Read the model definition and answer for the solid it produces. Units are mm, in the model's axes. A direction names the side the tool comes from. Give positions to 0.01 mm unless a question says otherwise; leave off trailing zeros. Loops run counter-clockwise (first coordinate to the right, second up) from the corner with the lowest first, then second, coordinate; pieces in that order, holes last. Notation, with made-up numbers: (-34.75, 89) - (0.25, 89) arc R23 ccw to (0.25, 97) - close; hole circle Ø8 at (21, 64). An arc over 180 degrees is marked (long way). Write item = value, one per line. Start each with the question number.
from build123d import *

# Parameters (mm, degrees)
SKETCH1_R                    = 150
BOSS_EXTRUDE1_DEPTH          = 75
CHAMFER1_SIZE                = 10
BOSS_EXTRUDE2_START          = -75
BOSS_EXTRUDE2_DEPTH          = 10
CHAMFER2_SIZE                = 7
BOSS_EXTRUDE3_DEPTH          = 9
BOSS_EXTRUDE4_DEPTH          = 3.5
CIRPATTERN1_COUNT            = 4
CIRPATTERN1_COPY_1_DEPTH     = 9
CIRPATTERN1_COPY_2_DEPTH     = 9
CIRPATTERN1_COPY_3_DEPTH     = 9
CIRPATTERN1_COPY_4_DEPTH     = 3.5
CIRPATTERN1_COPY_5_DEPTH     = 3.5
CIRPATTERN1_COPY_6_DEPTH     = 3.5
CHAMFER2_OF_CIRPATTERN1_SIZE = 7
CUT_EXTRUDE1_START           = -60
CUT_EXTRUDE1_DEPTH           = 60
SKETCH6_R                    = 110
BOSS_EXTRUDE5_DEPTH          = 9
BOSS_EXTRUDE5_TAPER          = 40
SKETCH7_R                    = 15
BOSS_EXTRUDE6_DEPTH          = 20


with BuildPart() as part:
    # Sketch1 → Boss-Extrude1 (new body)
    with BuildSketch(Plane(origin=(0, 0, 0), x_dir=(1, 0, 0), z_dir=(0, 1, 0))):
        with Locations(Location((0, 0, 0), (0, 0, 270))):
            Circle(SKETCH1_R)
    extrude(amount=BOSS_EXTRUDE1_DEPTH)

    # Chamfer1
    chamfer1_edges = [part.edges().sort_by_distance(p)[0] for p in [
        (0, 75, -150),
    ]]
    chamfer(chamfer1_edges, length=CHAMFER1_SIZE)

    # Sketch2 → Boss-Extrude2 (add)
    with BuildSketch(Plane(origin=(0, 75, 0), x_dir=(1, 0, 0), z_dir=(0, 1, 0)).offset(BOSS_EXTRUDE2_START)):
        with BuildLine():
            Line((-145.236875483, 37.5), (-195.236875483, 37.5))
            Line((-195.236875483, 37.5), (-195.236875483, -37.5))
            Line((-195.236875483, -37.5), (-145.236875483, -37.5))
            ThreePointArc((-145.236875483, -37.5), (-150, 0), (-145.236875483, 37.5))
        make_face()
    boss_extrude2 = extrude(amount=BOSS_EXTRUDE2_DEPTH)

    # Chamfer2
    chamfer2_edges = [part.edges().sort_by_distance(p)[0] for p in [
        (-195.236875483, 5, -37.5),
        (-195.236875483, 5, 37.5),
    ]]
    chamfer(chamfer2_edges, length=CHAMFER2_SIZE)

    # Sketch3 → Boss-Extrude3 (add)
    with BuildSketch(Plane.XY.offset(37.5)):
        Polygon((-145.236875483, 10), (-145.236875483, 65), (-170.556875483, 65), (-188.236875483, 10), align=None)
    boss_extrude3 = extrude(amount=-BOSS_EXTRUDE3_DEPTH)

    # Sketch4 → Boss-Extrude4 (add)
    with BuildSketch(Plane(origin=(0, 10, 0), x_dir=(1, 0, 0), z_dir=(0, 1, 0))):
        Polygon((-188.236875483, -21), (-183.04072306, -18), (-183.04072306, -12), (-188.236875483, -9), (-193.433027905, -12), (-193.433027905, -18), align=None)
    boss_extrude4 = extrude(amount=BOSS_EXTRUDE4_DEPTH)

    # Mirror1: Boss-Extrude3, Boss-Extrude4 across plane
    add(boss_extrude3.mirror(Plane.XY))
    add(boss_extrude4.mirror(Plane.XY))

    # CirPattern1: Boss-Extrude2, Boss-Extrude3, Boss-Extrude4 ×4 about axis
    cirpattern1_axis = Axis((0, 0, 0), (0, 1, 0))
    add([boss_extrude2.rotate(cirpattern1_axis, i * 360 / CIRPATTERN1_COUNT) for i in range(1, CIRPATTERN1_COUNT)])
    add([boss_extrude3.rotate(cirpattern1_axis, i * 360 / CIRPATTERN1_COUNT) for i in range(1, CIRPATTERN1_COUNT)])
    add([boss_extrude4.rotate(cirpattern1_axis, i * 360 / CIRPATTERN1_COUNT) for i in range(1, CIRPATTERN1_COUNT)])

    # CirPattern1 copy 1 sketch → CirPattern1 copy 1 (add)
    with BuildSketch(Plane(origin=(-37.5, 0, 0), x_dir=(0, 0, -1), z_dir=(-1, 0, 0))):
        Polygon((-145.236875483, -10), (-145.236875483, -65), (-170.556875483, -65), (-188.236875483, -10), align=None)
    extrude(amount=-CIRPATTERN1_COPY_1_DEPTH)

    # CirPattern1 copy 2 sketch → CirPattern1 copy 2 (add)
    with BuildSketch(Plane(origin=(0, 0, 37.5), x_dir=(-1, 0, 0), z_dir=(0, 0, 1))):
        Polygon((-145.236875483, -10), (-145.236875483, -65), (-170.556875483, -65), (-188.236875483, -10), align=None)
    extrude(amount=-CIRPATTERN1_COPY_2_DEPTH)

    # CirPattern1 copy 3 sketch → CirPattern1 copy 3 (add)
    with BuildSketch(Plane(origin=(37.5, 0, 0), x_dir=(0, 0, 1), z_dir=(1, 0, 0))):
        Polygon((-145.236875483, -10), (-145.236875483, -65), (-170.556875483, -65), (-188.236875483, -10), align=None)
    extrude(amount=-CIRPATTERN1_COPY_3_DEPTH)

    # CirPattern1 copy 4 sketch → CirPattern1 copy 4 (add)
    with BuildSketch(Plane(origin=(0, 10, 0), x_dir=(0, 0, -1), z_dir=(0, 1, 0))):
        Polygon((-188.236875483, 21), (-183.04072306, 18), (-183.04072306, 12), (-188.236875483, 9), (-193.433027905, 12), (-193.433027905, 18), align=None)
    extrude(amount=CIRPATTERN1_COPY_4_DEPTH)

    # CirPattern1 copy 5 sketch → CirPattern1 copy 5 (add)
    with BuildSketch(Plane(origin=(0, 10, 0), x_dir=(-1, 0, 0), z_dir=(0, 1, 0))):
        Polygon((-188.236875483, 21), (-183.04072306, 18), (-183.04072306, 12), (-188.236875483, 9), (-193.433027905, 12), (-193.433027905, 18), align=None)
    extrude(amount=CIRPATTERN1_COPY_5_DEPTH)

    # CirPattern1 copy 6 sketch → CirPattern1 copy 6 (add)
    with BuildSketch(Plane.ZX.offset(10)):
        Polygon((-188.236875483, 21), (-183.04072306, 18), (-183.04072306, 12), (-188.236875483, 9), (-193.433027905, 12), (-193.433027905, 18), align=None)
    extrude(amount=CIRPATTERN1_COPY_6_DEPTH)

    # Chamfer2 of CirPattern1
    chamfer2_of_cirpattern1_edges = [part.edges().sort_by_distance(p)[0] for p in [
        (-37.5, 5, 195.236875483),
        (37.5, 5, 195.236875483),
        (195.236875483, 5, 37.5),
        (195.236875483, 5, -37.5),
        (37.5, 5, -195.236875483),
        (-37.5, 5, -195.236875483),
    ]]
    chamfer(chamfer2_of_cirpattern1_edges, length=CHAMFER2_OF_CIRPATTERN1_SIZE)

    # Sketch5 → Cut-Extrude1 (cut)
    with BuildSketch(Plane(origin=(0, 75, 0), x_dir=(1, 0, 0), z_dir=(0, 1, 0)).offset(CUT_EXTRUDE1_START)):
        with BuildLine():
            ThreePointArc((-70, -121.24355653), (-98.994949366, -98.994949366), (-121.24355653, -70))
            Line((-121.24355653, -70), (-129.903810568, -75))
            ThreePointArc((-129.903810568, -75), (-106.066017178, -106.066017178), (-75, -129.903810568))
            Line((-75, -129.903810568), (-70, -121.24355653))
        make_face()
        with BuildLine():
            ThreePointArc((-65, -112.583302492), (-91.923881554, -91.923881554), (-112.583302492, -65))
            Line((-112.583302492, -65), (-121.24355653, -70))
            ThreePointArc((-121.24355653, -70), (-98.994949366, -98.994949366), (-70, -121.24355653))
            Line((-70, -121.24355653), (-65, -112.583302492))
        make_face()
    extrude(amount=CUT_EXTRUDE1_DEPTH, mode=Mode.SUBTRACT)

    # Sketch6 → Boss-Extrude5 (add)
    with BuildSketch(Plane(origin=(0, 75, 0), x_dir=(1, 0, 0), z_dir=(0, 1, 0))):
        Circle(SKETCH6_R)
    extrude(amount=BOSS_EXTRUDE5_DEPTH, taper=BOSS_EXTRUDE5_TAPER)

    # Sketch7 → Boss-Extrude6 (add)
    with BuildSketch(Plane(origin=(0, 84, 0), x_dir=(1, 0, 0), z_dir=(0, 1, 0))):
        with Locations(Location((0, 0, 0), (0, 0, 270))):
            Circle(SKETCH7_R)
    extrude(amount=BOSS_EXTRUDE6_DEPTH)


solid = part.part
1. For a pull along X with two mould halves and no side action, classify faces 5 (the flat face through (37.5, 32, -162)), 6 (the flat face through (-28.5, 38, -163)), 7 (the flat face through (-28.5, 37, 163)), 8 (the flat face through (-37.5, 32, -162)) as released by +X, released by -X, zero draft, split by the parting line, or undercut.
2. A tool of negligible diameter and unlimited length cuts with its end or side. For faces 1 (the flat face through (33, 65, -158)), 2 (the flat face through (-33, 65, -158)), 3 (the flat face through (162, 32, -37.5)), 4 (the flat face through (163, 37, 28.5)), from which of +Z, -Z, +X, -X, +Y, -Y can it reach the whole face along a straight path? Write none if from no direction.
3. A cutting plane is placed at A-A on x = 0. Give the vertices of the cut face in (y, z).
4. Given P1, Ø24, axis at x = -179, z = 8, coming from the +Y side; P2, Ø4, axis at x = -103, y = 67, coming from the -Z side; P3, Ø1, axis at y = 11.5, z = 14.5, coming from the -X side, each flat-ended and moving along its own axis, determine where each tip first touches the part or whether it passes through.
5. A cutting plane is placed at B-B on y = 97.5. Give the vertices of the cut face in (x, z), and give its area (3 significant figures).
6. Consider line 1 along X through (y, z) = (47, 174.5); line 2 along Y through (x, z) = (-73.5, 122); line 3 along X through (y, z) = (35.5, 2.5). Determine where each line is inside the solid, lowest interval first. Write a range as [from, to].
Reply:
q1.face_5 = released by +X
q1.face_6 = undercut
q1.face_7 = undercut
q1.face_8 = released by -X
q2.face_1 = -Z, +X, +Y
q2.face_2 = -Z, -X, +Y
q2.face_3 = -Z, +X, +Y, -Y
q2.face_4 = +X, +Y
q3.outline = (0, -195.24) - (10, -195.24) - (10, -150) - (65, -150) - (75, -140) - (75, -110) - (84, -102.45) - (84, -15) - (104, -15) - (104, 15) - (84, 15) - (84, 102.45) - (75, 110) - (75, 140) - (65, 150) - (10, 150) - (10, 195.24) - (0, 195.24) - close
q4.P1 = 13.5
q4.P2 = -109.63
q4.P3 = -193.43
q5.outline = circle Ø30 at (0, 0)
q5.area = 707 mm^2
q6.line_1 = [-37.5, -28.5], [28.5, 37.5]
q6.line_2 = [0, 15]
q6.line_3 = [-149.98, 149.98]
